Design review of the part shown in the three views and the two pictorial views. Dimensions are in mm from the part's minimum x, y and z. Coordinates: 2 decimals unless noted, no trailing zeros. Loops run counter-clockwise (first coordinate to the right, second up) from the corner with the lowest first, then second, coordinate; pieces in that order, holes last. Notation, with made-up numbers: (33.25, -17) -> (51.25, -17) arc R12 cw to (51.25, -11) -> close; hole circle Ø3 at (58, 72.5). An arc over 180 degrees is marked (long way). One line per item, written item: value. Start each with the question number.
1. Draft analysis for pull direction Z (two halves, no side actions). For the marked faces 1, 2, 3 and 4, state which applies: pulls with the +Z half, pulls with the -Z half, needs draft (parallel to the pull), parting line crosses it, or undercut.
2. Add section B-B on x = 55. Write out the cut boundary in (y, z), plus the area to 3 significant figures.
3. Add section C-C on z = 21.5. Write out the cut boundary in (x, y), plus the area to 3 significant figures.
4. Insertion check: pin 1 (5 mm diameter, centred on x = 65.5, z = 67, fed in from +Y). The pin has a flat end and moves straight along its axis. Give the tip position at first contact, or say it passes through.
5. For probe 1 along Z at (x, y) = (138.5, 38); probe 2 along Y at (x, z) = (25, 14), list the stretches that pass through material, from the lowest coordinate up.
6. Add section A-A on y = 28. Write out the cut boundary in (x, z), plus the area to 3 significant figures.
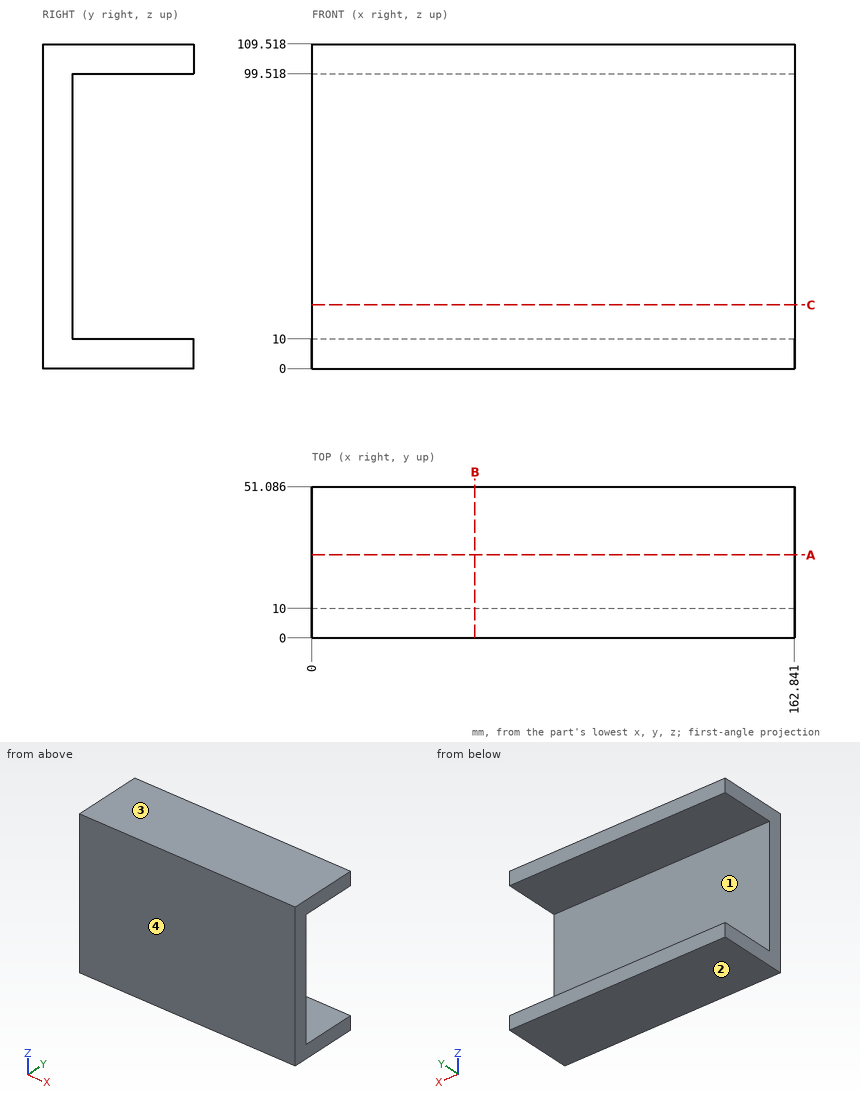
Worked answers:
1. face 1: undercut
1. face 2: pulls with the -Z half
1. face 3: pulls with the +Z half
1. face 4: needs draft
2. outline: (0, 0) -> (51.09, 0) -> (51.09, 10) -> (10, 10) -> (10, 99.52) -> (51.09, 99.52) -> (51.09, 109.52) -> (0, 109.52) -> close
2. area: 1,920 mm²
3. outline: (0, 0) -> (162.84, 0) -> (162.84, 10) -> (0, 10) -> close
3. area: 1,630 mm²
4. pin 1: stops at y = 10
5. probe 1: z = 0 to 10, 99.52 to 109.52
5. probe 2: y = 0 to 10
6. outline: (0, 0) -> (162.84, 0) -> (162.84, 10) -> (0, 10) -> close; (0, 99.52) -> (162.84, 99.52) -> (162.84, 109.52) -> (0, 109.52) -> close
6. area: 3,260 mm²
